Verification items for the finished model (mm, model axes). Give positions to 0.01 mm unless a question says otherwise; leave off trailing zeros. Write each loop counter-clockwise with the first axis right and the second up, starting at its lowest first coordinate (ties: lowest second). Pieces come first, ordered by that corner, then holes. Notation, with made-up numbers: (34.25, 6.5) -> (48.25, 6.5) arc R15 cw to (48.25, 16.5) -> close; hole circle Ø11 at (36, 71.25). An arc over 180 degrees is marked (long way). Answer as CSV lines item,"result".
```python
from build123d import *

# Parameters (mm, degrees)
SKETCH1_R           = 73.025
BOSS_EXTRUDE1_DEPTH = 6.35
CUT_EXTRUDE2_START  = -6.35
SKETCH2_R           = 4.7625
SKETCH2_R_2         = 6.35
CUT_EXTRUDE2_DEPTH  = 6.35
SKETCH3_R           = 1.75
SKETCH3_R_2         = 1.5
CUT_EXTRUDE3_DEPTH  = 10
CUT_EXTRUDE7_DEPTH  = 83.240634572
FILLET1_R           = 2.54


with BuildPart() as part:
    # Sketch1 → Boss-Extrude1 (new body)
    with BuildSketch(Plane(origin=(0, 0, 0), x_dir=(1, 0, 0), z_dir=(0, 1, 0))):
        with Locations(Location((0, 0, 0), (0, 0, 270))):
            Circle(SKETCH1_R)
    extrude(amount=BOSS_EXTRUDE1_DEPTH)

    # Sketch2 → Cut-Extrude2 (cut)
    with BuildSketch(Plane(origin=(0, 6.35, 0), x_dir=(1, 0, 0), z_dir=(0, 1, 0)).offset(CUT_EXTRUDE2_START)):
        with BuildLine():
            ThreePointArc((61.150770614, -23.195291499), (0, -37.290063688), (-61.150770614, -23.195291499))
            ThreePointArc((-61.150770614, -23.195291499), (-66.917906968, -19.630921399), (-71.53671875, -14.667941079))
            ThreePointArc((-71.53671875, -14.667941079), (0, -73.025), (71.53671875, -14.667941079))
            ThreePointArc((71.53671875, -14.667941079), (66.917906968, -19.630921399), (61.150770614, -23.195291499))
        make_face()
        with BuildLine():
            ThreePointArc((-61.150770614, 23.195291499), (0, 37.290063688), (61.150770614, 23.195291499))
            ThreePointArc((61.150770614, 23.195291499), (66.917906968, 19.630921399), (71.53671875, 14.667941079))
            ThreePointArc((71.53671875, 14.667941079), (0, 73.025), (-71.53671875, 14.667941079))
            ThreePointArc((-71.53671875, 14.667941079), (-66.917906968, 19.630921399), (-61.150770614, 23.195291499))
        make_face()
        with Locations(Location((-50.8, 0, 0), (0, 0, 270))):
            Circle(SKETCH2_R)
        with Locations(Location((50.8, 0, 0), (0, 0, 270))):
            Circle(SKETCH2_R)
        with Locations(Location((0, 0, 0), (0, 0, 270))):
            Circle(SKETCH2_R_2)
    extrude(amount=CUT_EXTRUDE2_DEPTH, mode=Mode.SUBTRACT)

    # Sketch3 → Cut-Extrude3 (cut)
    # profile 1 of 8: a face of its own
    with BuildSketch(Plane.XZ):
        with Locations(Location((-9, 8.5, 0), (0, 0, 270))):
            Circle(SKETCH3_R)
        with Locations((-9, 8.5)):
            Circle(SKETCH3_R_2, mode=Mode.SUBTRACT)
    # profile 2 of 8: a face of its own
    with BuildSketch(Plane.XZ):
        with Locations((-9, 8.5)):
            Circle(SKETCH3_R_2)
    # profile 3 of 8: a face of its own
    with BuildSketch(Plane.XZ):
        with Locations(Location((-9, -24.5, 0), (0, 0, 270))):
            Circle(SKETCH3_R)
        with Locations((-9, -24.5)):
            Circle(SKETCH3_R_2, mode=Mode.SUBTRACT)
    # profile 4 of 8: a face of its own
    with BuildSketch(Plane.XZ):
        with Locations((-9, -24.5)):
            Circle(SKETCH3_R_2)
    # profile 5 of 8: a face of its own
    with BuildSketch(Plane.XZ):
        with Locations(Location((9, -24.5, 0), (0, 0, 270))):
            Circle(SKETCH3_R)
        with Locations((9, -24.5)):
            Circle(SKETCH3_R_2, mode=Mode.SUBTRACT)
    # profile 6 of 8: a face of its own
    with BuildSketch(Plane.XZ):
        with Locations((9, -24.5)):
            Circle(SKETCH3_R_2)
    # profile 7 of 8: a face of its own
    with BuildSketch(Plane.XZ):
        with Locations(Location((9, 8.5, 0), (0, 0, 270))):
            Circle(SKETCH3_R)
        with Locations((9, 8.5)):
            Circle(SKETCH3_R_2, mode=Mode.SUBTRACT)
    # profile 8 of 8: a face of its own
    with BuildSketch(Plane.XZ):
        with Locations((9, 8.5)):
            Circle(SKETCH3_R_2)
    extrude(amount=-CUT_EXTRUDE3_DEPTH, mode=Mode.SUBTRACT)

    # Sketch5 → Cut-Extrude7 (cut, through all)
    with BuildSketch(Plane(origin=(0, 6.35, 0), x_dir=(1, 0, 0), z_dir=(0, 1, 0))):
        with BuildLine():
            add(Edge.make_bspline(
                [(-61.150770614, -23.195291499), (0, -13.284835877), (61.150770614, -23.195291499)],
                knots=[0, 0, 0, 1, 1, 1], degree=2))
            ThreePointArc((-61.150770614, -23.195291499), (0, -37.290063688), (61.150770614, -23.195291499))
        make_face()
    extrude(amount=-CUT_EXTRUDE7_DEPTH, mode=Mode.SUBTRACT)

    # Fillet1
    fillet1_edges = [part.edges().sort_by_distance(p)[0] for p in [
        (61.150770614, 3.175, 23.195291499),
        (-61.150770614, 3.175, 23.195291499),
    ]]
    fillet(fillet1_edges, radius=FILLET1_R)


solid = part.part
```
1) Draft check along X on faces 1 (the flat face through (1, 6.35, -8)), 2 (the cylindrical face through (-7.5, 3.1, 7.6)), 3 (the cylindrical face through (66.844, 3.131, -19.691)). Enter one of: +X half, -X half, draft (parallel to the pull), parting line (faces both ways), or undercut.
Reported:
face 1,"draft"
face 2,"undercut"
face 3,"+X half"
2) Depth check by flat-ended pin: pin 1 (2 mm diameter, centred on y = 3, z = -16.5, fed in from +X); pin 2 (12.5 mm diameter, centred on x = 50.8, z = 0, fed in from -Y); pin 3 (1 mm diameter, centred on y = 1, z = -12, fed in from +X). Enter the tip coordinate at first touch or a pass-through.
Reported:
pin 1,"x = 70.92"
pin 2,"y = 0"
pin 3,"x = 72.11"
3) Scan lines: line 1 along X through (y, z) = (3.75, 8.5); line 2 along X through (y, z) = (4.75, -25); line 3 along X through (y, z) = (0.5, 1). Record each from-to range of solid material in increasing order.
Reported:
line 1,"-72.53 to -10.75, -7.25 to 7.25, 10.75 to 72.53"
line 2,"-57.3 to -10.68, -7.32 to 7.32, 10.68 to 57.3"
line 3,"-73.02 to -55.46, -46.14 to -6.27, 6.27 to 46.14, 55.46 to 73.02"
4) Section check A-A (z = 0). State how many separate pieces and enclosed holes the cut face has, and give its area (3 significant figures).
Reported:
separate pieces,"4"
enclosed holes,"0"
area,"726 mm²"
5) Section check B-B (z = -24.5). Record the boundary of the cut face in (x, y).
Reported:
outline,"(-58.39, 0) -> (-10.75, 0) -> (-10.75, 6.35) -> (-58.39, 6.35) -> close; (-7.25, 0) -> (7.25, 0) -> (7.25, 6.35) -> (-7.25, 6.35) -> close; (10.75, 0) -> (58.39, 0) -> (58.39, 6.35) -> (10.75, 6.35) -> close"
